The model under review builds one solid part; all positions refer to its coordinate system, in mm. Coordinates: 2 decimals unless noted, no trailing zeros. Order: outer loops, then holes, each group sorted by start corner. A loop starts at its lowest first (then second) coordinate and runs counter-clockwise, first axis right, second up. Notation, with made-up numbers: M 36.25,80.25 L 72.25,80.25 A9 cw 72.25,90.25 Z; hole C 30,-14 d1. An arc over 180 degrees is marked long. One line per item, written item: value.
Autodesk Fusion 360 part; units mm, degrees
sketch "Sketch2" plane through (0, 0, 0) normal (0, 1, 0) x (1, 0, 0)
  line L0 (-34.5, -4.5) -> (34.5, -4.5)
  line L1 (34.5, -4.5) -> (34.5, 4.5)
  line L2 (34.5, 4.5) -> (-34.5, 4.5)
  line L3 (-34.5, 4.5) -> (-34.5, -4.5)
  line L4 (-34.5, -4.5) -> (34.5, 4.5) construction
  line L5 (34.5, -4.5) -> (-34.5, 4.5) construction
  circle A0 centre (0, 0) radius 2.5
  dimension "d1" = 69
  dimension "d2" = 9
  dimension "d3" = 5
extrude "Extrude1" add sketch "Sketch2" along normal blind 2 contours L0 L1 L2 L3 | A0 makes body 1
sketch "Sketch3" plane through (0, 2, 0) normal (0, 1, 0) x (-1, 0, 0)
  line L0 (34.5, -4.5) -> (34.5, 4.5)
  line L1 (34.5, 4.5) -> (-34.5, 4.5)
  line L2 (-34.5, 4.5) -> (-34.5, -4.5)
  line L3 (-34.5, -4.5) -> (34.5, -4.5)
  circle A0 centre (0, 0) radius 2.5
  circle A1 centre (0, 0) radius 2.5
extrude "Extrude3" add sketch "Sketch3" along normal blind 6 contours A0 A1 bodies 1
fillet "Fillet3" radius 2 1 edges at (2.3308, 2, 0.904) on bodies 1
fillet "Fillet4" radius 2 1 edges at (2.3308, 8, -0.904) on bodies 1
chamfer "Chamfer2" distance 2 angle 45 4 edges at (34.5, 1, 4.5) (34.5, 1, -4.5) (-34.5, 1, -4.5) (-34.5, 1, 4.5) on bodies 1
copy_body "Body->Comp1" bodies 1 removing the originals makes body 2 in component "spring"
component "spring" placed x (1, 0, 0) y (0, 1, 0) z (0, 0, 1) at (0, 0, 0)
equation "d4 = spring_thickness"
equation "d15 = post_length"
equation "spring_thickness = 2 mm"
equation "post_length = 6 mm"
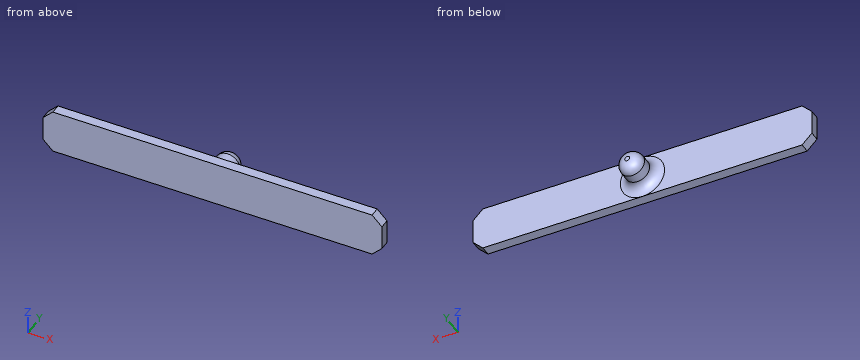
(1) Insertion check: pin 1 Ø2 at (y, z) = (6, -1.5) entering from -X; pin 2 Ø2.5 at (x, z) = (14, 1.5) entering from +Y. Each pin has a flat end and moves straight along its axis. Give the tip position at first contact, or say it passes through.
Geometry results:
pin 1: stops at x = -2.45
pin 2: stops at y = 2
(2) We need section B-B, the plane y = 3. State the section outline as (x, z) points, plus the area to 3 significant figures.
Geometry results:
outline: C 0,0 d5.54
area: 24.1 mm2
(3) For L1, parallel to Y at x = 17, z = -3.75; L2, parallel to X at y = 0.5, z = -3; L3, parallel to X at y = 0.5, z = 3.5, list the stretches that pass through material, from the lowest coordinate up.
Geometry results:
L1: y = 0 to 2
L2: x = -34 to 34
L3: x = -33.5 to 33.5
(4) We need section A-A, the plane x = 24.5. State the section outline as (y, z) points, plus the area to 3 significant figures.
Geometry results:
outline: M 0,-4.5 L 2,-4.5 L 2,4.5 L 0,4.5 Z
area: 18.0 mm2
